from build123d import *

# Parameters (mm, degrees)
SKETCH_1_W      = 25
SKETCH_1_H      = 40
SKETCH_1_R      = 1.5
EXTRUDE_1_DEPTH = 4
FILLET_1_R      = 5


with BuildPart() as part:
    # 草图1 → 凸台-拉伸1 (new body)
    with BuildSketch(Plane.XY):
        Rectangle(SKETCH_1_W, SKETCH_1_H)
        with Locations((-7.5, 15)):
            Circle(SKETCH_1_R, mode=Mode.SUBTRACT)
        with Locations((7.5, 15)):
            Circle(SKETCH_1_R, mode=Mode.SUBTRACT)
        with Locations((-7.5, -15)):
            Circle(SKETCH_1_R, mode=Mode.SUBTRACT)
        with Locations((7.5, -15)):
            Circle(SKETCH_1_R, mode=Mode.SUBTRACT)
        with Locations((-7.5, 7.5)):
            Circle(SKETCH_1_R, mode=Mode.SUBTRACT)
        with Locations((7.5, 7.5)):
            Circle(SKETCH_1_R, mode=Mode.SUBTRACT)
        with Locations((7.5, -7.5)):
            Circle(SKETCH_1_R, mode=Mode.SUBTRACT)
        with Locations((-7.5, -7.5)):
            Circle(SKETCH_1_R, mode=Mode.SUBTRACT)
    extrude(amount=EXTRUDE_1_DEPTH)

    # 圆角1
    fillet_1_edges = [part.edges().sort_by_distance(p)[0] for p in [
        (12.5, -20, 2),
        (-12.5, -20, 2),
        (-12.5, 20, 2),
        (12.5, 20, 2),
    ]]
    fillet(fillet_1_edges, radius=FILLET_1_R)


solid = part.part
Input: part model. Units: mm. Frame: model coordinates. Coordinates: 2 decimals unless noted, no trailing zeros. Loops run counter-clockwise (first coordinate to the right, second up) from the corner with the lowest first, then second, coordinate; pieces in that order, holes last. Notation, with made-up numbers: (82, -17.5) - (109, -17.5) arc R32 ccw to (109, 8.5) - close; hole circle Ø5 at (79.5, -24). An arc over 180 degrees is marked (long way). Answer in a Markdown table with one row per item. Add a question column.
Item 1: Section query A-A on z = 2.2. State how many separate pieces and enclosed holes the cut face has, then the cut area to 3 significant figures.
Item 2: Contact query for flat-ended pins moving along their axis: P1, Ø2.5, axis at x = -7.5, y = -15, coming from the -Z side; P2, Ø1.5, axis at x = -8.5, y = 15.5, coming from the +Z side. Output: stop coordinate, or through.
Item 3: Line query: line 1 along Y through (x, z) = (-7.5, 1.7); line 2 along X through (y, z) = (8.5, 0.95); line 3 along X through (y, z) = (-16, 2.05). Output: solid intervals per line, ascending. Write a range as [from, to].
Item 4: Section query B-B on y = 7. Return the cut outline in (x, z), then the cut area to 3 significant figures.
Item 5: Section query C-C on x = -9.5. Return the cut outline in (y, z), then the cut area to 3 significant figures.
Item 6: Mould query, pull axis Y, two halves, no side actions, for faces 1 (the cylindrical face through (-11.07, -18.5, 2.03)), 2 (the flat face through (0, 0, 0)), 3 (the cylindrical face through (6.3, 6.6, 2)). Classes: released by +Y, released by -Y, zero draft, split by the parting line, or undercut.
Recorded:
| question | item | result |
|---|---|---|
| 1 | separate pieces | 1 |
| 1 | enclosed holes | 8 |
| 1 | area | 922 mm^2 |
| 2 | P1 | through |
| 2 | P2 | z = 4 |
| 3 | line 1 | [-20, -16.5], [-13.5, -9], [-6, 6], [9, 13.5], [16.5, 20] |
| 3 | line 2 | [-12.5, -8.62], [-6.38, 6.38], [8.62, 12.5] |
| 3 | line 3 | [-12.4, -8.62], [-6.38, 6.38], [8.62, 12.4] |
| 4 | outline | (-12.5, 0) - (-8.91, 0) - (-8.91, 4) - (-12.5, 4) - close; (-6.09, 0) - (6.09, 0) - (6.09, 4) - (-6.09, 4) - close; (8.91, 0) - (12.5, 0) - (12.5, 4) - (8.91, 4) - close |
| 4 | area | 77.4 mm^2 |
| 5 | outline | (-19.58, 0) - (19.58, 0) - (19.58, 4) - (-19.58, 4) - close |
| 5 | area | 157 mm^2 |
| 6 | face 1 | released by -Y |
| 6 | face 2 | zero draft |
| 6 | face 3 | undercut |
